The listing builds one solid part. Answer for the finished solid, in the listing's coordinates (mm). Face numbers are marked on the shaded views. A direction names the side the tool comes from. Coordinates: 2 decimals unless noted, no trailing zeros. Loops run counter-clockwise (first coordinate to the right, second up) from the corner with the lowest first, then second, coordinate; pieces in that order, holes last. Notation, with made-up numbers: (46, -39.75) - (90, -39.75) arc R28 cw to (90, -8.75) - close; hole circle Ø1 at (89, 85.5). An arc over 180 degrees is marked (long way). Put each result on its own line as item: value.
```python
from build123d import *

# Parameters (mm, degrees)
SKETCH4_R                    = 4
BOSS_EXTRUDE1_DEPTH          = 0.5
SKETCH5_R                    = 2
BOSS_EXTRUDE2_DEPTH          = 10.5
CHAMFER1_SIZE                = 0.5
CIRPATTERN1_COUNT            = 3
CHAMFER1_OF_CIRPATTERN1_SIZE = 0.5
BOSS_EXTRUDE3_DEPTH          = 7.5
SKETCH7_R                    = 0.75
CUT_EXTRUDE1_DEPTH           = 2
CUT_EXTRUDE2_DEPTH           = 34.068111528
CHAMFER2_SIZE                = 0.2
CHAMFER3_SIZE                = 0.5
CIRPATTERN2_COUNT            = 3
CHAMFER2_OF_CIRPATTERN2_SIZE = 0.2
CHAMFER3_OF_CIRPATTERN2_SIZE = 0.5
CHAMFER4_SIZE                = 1
FILLET1_R                    = 1


with BuildPart() as part:
    # Sketch3 → Revolve1 (revolve)
    with BuildSketch(Plane(origin=(0, 0, 0), x_dir=(0, 0, -1), z_dir=(1, 0, 0)), mode=Mode.PRIVATE) as revolve1_sk:
        Polygon((1, 13.6), (1, 12), (2.5, 12), (2.5, 10), (5.5, 10), (5.5, 21.5), (1.5, 21.5), (1.5, 20), (0, 20), (0, 13.6), align=None)
    revolve(revolve1_sk.sketch.rotate(Axis((0, 0, 0), (0, 0, -1)), 90), axis=Axis((0, 0, 0), (0, 0, -1)))

    # Sketch4 → Boss-Extrude1 (add)
    with BuildSketch(Plane(origin=(0, 0, -5.5), x_dir=(-1, 0, 0), z_dir=(0, 0, -1))):
        with Locations(Location((0, 16.8, 0), (0, 0, 180))):
            Circle(SKETCH4_R)
    boss_extrude1 = extrude(amount=BOSS_EXTRUDE1_DEPTH)

    # Sketch5 → Boss-Extrude2 (add)
    with BuildSketch(Plane(origin=(0, 0, -6), x_dir=(-1, 0, 0), z_dir=(0, 0, -1))):
        with Locations(Location((0, 16.8, 0), (0, 0, 180))):
            Circle(SKETCH5_R)
    boss_extrude2 = extrude(amount=BOSS_EXTRUDE2_DEPTH)

    # Chamfer1
    chamfer1_edges = [part.edges().sort_by_distance(p)[0] for p in [
        (-2, 16.8, -16.5),
    ]]
    chamfer(chamfer1_edges, length=CHAMFER1_SIZE)

    # CirPattern1: Boss-Extrude1, Boss-Extrude2 ×3 about axis
    cirpattern1_axis = Axis((0, 0, 0), (0, 0, 1))
    add([boss_extrude1.rotate(cirpattern1_axis, i * 360 / CIRPATTERN1_COUNT) for i in range(1, CIRPATTERN1_COUNT)])
    add([boss_extrude2.rotate(cirpattern1_axis, i * 360 / CIRPATTERN1_COUNT) for i in range(1, CIRPATTERN1_COUNT)])

    # Chamfer1 of CirPattern1
    chamfer1_of_cirpattern1_edges = [part.edges().sort_by_distance(p)[0] for p in [
        (-13.549226784, -10.132050808, -16.5),
        (15.549226784, -6.667949192, -16.5),
    ]]
    chamfer(chamfer1_of_cirpattern1_edges, length=CHAMFER1_OF_CIRPATTERN1_SIZE)

    # Sketch6 → Boss-Extrude3 (add)
    with BuildSketch(Plane(origin=(0, 0, -5.5), x_dir=(-1, 0, 0), z_dir=(0, 0, -1))):
        with BuildLine():
            ThreePointArc((-4.561681399, -8.89893605), (-6.703398823, -14.60024061), (-11.755277198, -18.001762636))
            ThreePointArc((-11.755277198, -18.001762636), (0, -21.5), (11.755277198, -18.001762636))
            ThreePointArc((11.755277198, -18.001762636), (6.703398823, -14.60024061), (4.561681399, -8.89893605))
            ThreePointArc((4.561681399, -8.89893605), (0, -10), (-4.561681399, -8.89893605))
        make_face()
    boss_extrude3 = extrude(amount=BOSS_EXTRUDE3_DEPTH)

    # Sketch7 → Cut-Extrude1 (cut)
    with BuildSketch(Plane(origin=(0, 0, -13), x_dir=(-1, 0, 0), z_dir=(0, 0, -1))):
        with BuildLine():
            Line((-3.105828541, -11.591109915), (-4.658742812, -17.386664873))
            ThreePointArc((-4.658742812, -17.386664873), (0, -18), (4.658742812, -17.386664873))
            Line((4.658742812, -17.386664873), (3.105828541, -11.591109915))
            ThreePointArc((3.105828541, -11.591109915), (0, -12), (-3.105828541, -11.591109915))
        make_face()
        with Locations((0, -15)):
            Circle(SKETCH7_R, mode=Mode.SUBTRACT)
    cut_extrude1 = extrude(amount=-CUT_EXTRUDE1_DEPTH, mode=Mode.SUBTRACT)

    # Sketch7<3> → Cut-Extrude2 (cut, through all)
    with BuildSketch(Plane(origin=(0, 0, -13), x_dir=(-1, 0, 0), z_dir=(0, 0, -1))):
        with BuildLine():
            ThreePointArc((0.75, -15), (0.530330086, -14.469669914), (0, -14.25))
            Line((0, -14.25), (0, -15.75))
            ThreePointArc((0, -15.75), (0.530330086, -15.530330086), (0.75, -15))
        make_face()
        with BuildLine():
            Line((0, -15.75), (0, -14.25))
            ThreePointArc((0, -14.25), (-0.75, -15), (0, -15.75))
        make_face()
    cut_extrude2 = extrude(amount=-CUT_EXTRUDE2_DEPTH, mode=Mode.SUBTRACT)

    # Chamfer2
    chamfer2_edges = [part.edges().sort_by_distance(p)[0] for p in [
        (0, -15.75, -11),
    ]]
    chamfer(chamfer2_edges, length=CHAMFER2_SIZE)

    # Chamfer3
    chamfer3_edges = [part.edges().sort_by_distance(p)[0] for p in [
        (0, -12, -13),
        (3.882285677, -14.488887394, -13),
        (0, -18, -13),
        (-3.882285677, -14.488887394, -13),
    ]]
    chamfer(chamfer3_edges, length=CHAMFER3_SIZE)

    # CirPattern2: Boss-Extrude3, Cut-Extrude1, Cut-Extrude2 ×3 about axis
    cirpattern2_axis = Axis((0, 0, 0), (0, 0, 1))
    add([boss_extrude3.rotate(cirpattern2_axis, i * 360 / CIRPATTERN2_COUNT) for i in range(1, CIRPATTERN2_COUNT)])
    add([cut_extrude1.rotate(cirpattern2_axis, i * 360 / CIRPATTERN2_COUNT) for i in range(1, CIRPATTERN2_COUNT)], mode=Mode.SUBTRACT)
    add([cut_extrude2.rotate(cirpattern2_axis, i * 360 / CIRPATTERN2_COUNT) for i in range(1, CIRPATTERN2_COUNT)], mode=Mode.SUBTRACT)

    # Chamfer2 of CirPattern2
    chamfer2_of_cirpattern2_edges = [part.edges().sort_by_distance(p)[0] for p in [
        (13.63990011, 7.875, -11),
        (-13.63990011, 7.875, -11),
    ]]
    chamfer(chamfer2_of_cirpattern2_edges, length=CHAMFER2_OF_CIRPATTERN2_SIZE)

    # Chamfer3 of CirPattern2
    chamfer3_of_cirpattern2_edges = [part.edges().sort_by_distance(p)[0] for p in [
        (10.392304845, 6, -13),
        (10.606601718, 10.606601718, -13),
        (15.588457268, 9, -13),
        (14.488887394, 3.882285677, -13),
        (-10.392304845, 6, -13),
        (-14.488887394, 3.882285677, -13),
        (-15.588457268, 9, -13),
        (-10.606601718, 10.606601718, -13),
    ]]
    chamfer(chamfer3_of_cirpattern2_edges, length=CHAMFER3_OF_CIRPATTERN2_SIZE)

    # Chamfer4
    chamfer4_edges = [part.edges().sort_by_distance(p)[0] for p in [
        (-20, 0, 0),
    ]]
    chamfer(chamfer4_edges, length=CHAMFER4_SIZE)

    # Fillet1
    # the kernel refuses this fillet: 1 mm, written as the material it takes off along each edge
    with BuildSketch(Plane(origin=(21.467622355, -1.179487364, -5.5), x_dir=(0.006387197521753026, 0.9999796016458627, 0), z_dir=(0, 0, -1)), Plane(origin=(-9.712345156, 19.18125, -5.5), x_dir=(-0.8692013370524359, -0.4944583255101058, 0), z_dir=(0, 0, -1)), Plane(origin=(-11.755277198, -18.001762636, -5.5), x_dir=(0.8628141395306828, -0.5055212761357604, 0), z_dir=(0, 0, -1))) as fillet1_piece_1:
        with BuildLine():
            CenterArc((2.036209541, -0.998824096), FILLET1_R, 87.221143718, 125.050734124)
            ThreePointArc((1.190685537, -1.532761506), (0.632617432, -0.737424909), (0, 0))
            ThreePointArc((0, 0), (1.04234536, 0.025281931), (2.084690721, 0))
        make_face()
    extrude(amount=12.711726802, mode=Mode.SUBTRACT)
    with BuildSketch(Plane(origin=(9.987545385, 0.49893605, -5.5), x_dir=(0.917317562643698, 0.39815636283428313, 0), z_dir=(0, 0, -1)), Plane(origin=(-5.425863987, 8.4, -5.5), x_dir=(-0.8034723062147525, 0.5953421311699238, 0), z_dir=(0, 0, -1)), Plane(origin=(-4.561681399, -8.89893605, -5.5), x_dir=(-0.113845256428944, -0.9934984940042073, 0), z_dir=(0, 0, -1))) as fillet1_piece_2:
        with BuildLine():
            CenterArc((1.346819148, -0.99794128), FILLET1_R, 93.677145319, 99.571657965)
            ThreePointArc((0.373435102, -1.22712134), (0.20641295, -0.607567006), (0, 0))
            ThreePointArc((0, 0), (0.641342451, -0.020587199), (1.282684903, 0))
        make_face()
    extrude(amount=10.706712257, mode=Mode.SUBTRACT)
    with BuildSketch(Plane(origin=(5.425863987, 8.4, -5.5), x_dir=(0.8034723062147446, 0.5953421311699345, 0), z_dir=(0, 0, -1)), Plane(origin=(-9.987545385, 0.49893605, -5.5), x_dir=(-0.9173175626437023, 0.3981563628342732, 0), z_dir=(0, 0, -1)), Plane(origin=(4.561681399, -8.89893605, -5.5), x_dir=(0.11384525642895783, -0.9934984940042058, 0), z_dir=(0, 0, -1))) as fillet1_piece_3:
        with BuildLine():
            CenterArc((1.346819148, 0.99794128), FILLET1_R, 166.751196715, 99.571657965)
            ThreePointArc((0.373435102, 1.22712134), (0.20641295, 0.607567006), (0, 0))
            ThreePointArc((0, 0), (0.641342451, 0.020587199), (1.282684903, 0))
        make_face()
    extrude(amount=10.706712257, mode=Mode.SUBTRACT)
    with BuildSketch(Plane(origin=(9.712345156, 19.18125, -5.5), x_dir=(0.8692013370524442, -0.49445832551009133, 0), z_dir=(0, 0, -1)), Plane(origin=(-21.467622355, -1.179487364, -5.5), x_dir=(-0.006387197521764941, 0.9999796016458625, 0), z_dir=(0, 0, -1)), Plane(origin=(11.755277198, -18.001762636, -5.5), x_dir=(-0.8628141395306764, -0.5055212761357711, 0), z_dir=(0, 0, -1))) as fillet1_piece_4:
        with BuildLine():
            CenterArc((2.036209541, 0.998824096), FILLET1_R, 147.728122158, 125.050734124)
            ThreePointArc((1.190685537, 1.532761506), (0.632617432, 0.737424909), (0, 0))
            ThreePointArc((0, 0), (1.04234536, -0.025281931), (2.084690721, 0))
        make_face()
    extrude(amount=12.711726802, mode=Mode.SUBTRACT)


solid = part.part
```
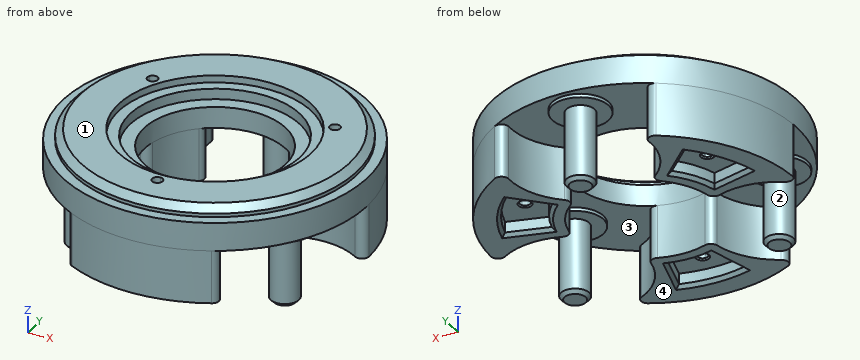
1) The part is cut by section A-A (z = -13.75). Give the vertices of the cut face in (x, y), and give its area (3 significant figures).
Found:
outline: circle Ø4 at (-14.55, -8.4); circle Ø4 at (0, 16.8); circle Ø4 at (14.55, -8.4)
area: 37.7 mm^2
2) For the marked faces 1 and 2, determine the directions among +Z, -Z, +X, -X, +Y, -Y from which every point of the face is accessible in a straight line to the end or side of a thin tool.
Found:
face 1: +Z, +X, -X, +Y, -Y
face 2: -Z
3) Straight lines are drawn through the part: L1, parallel to Y at x = 0, z = -1.75; L2, parallel to Y at x = 0, z = -1.3; L3, parallel to Z at x = 9.5, y = -18. For each, find the intervals that lie inside material, in ascending order. Write a range as [from, to].
Found:
L1: y = [-21.5, -15.75], [-14.25, -12], [12, 21.5]
L2: y = [-20, -15.75], [-14.25, -12], [12, 20]
L3: z = [-13, -1.5]
4) For a pull along Y with two mould halves and no side action, classify the marked faces 3 and 4 as pulls with the +Y half, pulls with the -Y half, needs draft (parallel to the pull), parting line crosses it, or undercut.
Found:
face 3: undercut
face 4: needs draft
5) Each of these flat-tipped pins is pushed along its axis until it touches: pin 1 (1 mm diameter, centred on x = -8, z = -3.5, fed in from -Y); pin 2 (4.5 mm diameter, centred on x = 11, y = 9, fed in from -Z); pin 3 (4 mm diameter, centred on x = -4.5, y = 17, fed in from -Z); pin 4 (19 mm diameter, centred on x = 0, y = 0, fed in from +Z). Where does it stop, or does it pass through?
Found:
pin 1: stops at y = -20.15
pin 2: stops at z = -13
pin 3: stops at z = -6
pin 4: passes through
